Source: CAD feature listing. Evaluate the final solid. Frame: model axes, mm. Coordinates: 2 decimals unless noted, no trailing zeros. Loops run counter-clockwise (first coordinate to the right, second up) from the corner with the lowest first, then second, coordinate; pieces in that order, holes last.
Autodesk Inventor part; units mm, degrees
ref_plane "YZ Plane" through (0, 0, 0) normal (1, 0, 0) x (0, 1, 0)
ref_plane "XZ Plane" through (0, 0, 0) normal (0, 1, 0) x (-1, 0, 0)
ref_plane "XY Plane" through (0, 0, 0) normal (0, 0, 1) x (1, 0, 0)
sketch "Sketch1" plane through (0, 0, 0) normal (0, 0, 1) x (1, 0, 0)
  line L0 (0, 0) -> (10, 0)
  line L1 (10, 0) -> (10, 40)
  line L2 (10, 40) -> (0, 40)
  line L3 (0, 40) -> (0, 0)
  dimension "d0" = 10
  dimension "d1" = 40
extrude "Extrusion1" add sketch "Sketch1" along normal blind 1
sketch "Sketch2" plane through (0, 0, 1) normal (0, 0, 1) x (1, 0, 0)
  line L0 (10, 40) -> (0, 40)
  line L1 (0, 40) -> (5, 40)
  line L2 (5, 40) -> (5, 35)
  circle A0 centre (5, 35) radius 2.5
  line L3 (0, 0) -> (1, 0)
  line L4 (1, 0) -> (5, 0)
  line L5 (0, 0) -> (10, 0)
  line L6 (5, 0) -> (5, 5)
  circle A1 centre (5, 5) radius 2.5
  dimension "d4" = 5
  dimension "d5" = 5
  dimension "d6" = 5
  dimension "d7" = 1
  dimension "d8" = 4
  dimension "d9" = 5
  dimension "d10" = 5
extrude "Extrusion2" cut sketch "Sketch2" against normal blind 1
sketch "Sketch3" plane through (0, 0, 1) normal (0, 0, 1) x (1, 0, 0)
  circle A0 centre (4.7625, 4.7625) radius 4
  point P0 (0, 0)
  dimension "d13" = 8
properties part number "crank"
Q1. Draft query along X for faces 1 (the cylindrical face through (7.385, 35.751, 0.507)), 2 (the flat face through (0, 20.3, 0.5)), 3 (the flat face through (5, 20, 0)). Return one class per face: released by +X, released by -X, zero draft, split by the parting line, or undercut.
Q2. Section query C-C on z = 0.6. Return the cut outline in (x, y), then the cut area to 3 significant figures.
Q3. Section query A-A on x = 5. Return the cut outline in (y, z), then the cut area to 3 significant figures.
Q4. Material intervals for line 1 along Y through (x, z) = (5, 0.6); line 2 along X through (y, z) = (5, 0.55); line 3 along Y through (x, z) = (6, 0.15), sorted ascending.
Q5. First-contact query: pin 1 Ø4 at (x, y) = (5, 5) entering from -Z. Flat tip, straight axial feed; report the tip coordinate or a pass-through.
Q6. Section query B-B on y = 35. Return the cut outline in (x, z), then the cut area to 3 significant figures.
Q7. Section query D-D on y = 6.5. Return the cut outline in (x, z).
Resolved:
1. face 1: undercut
1. face 2: released by -X
1. face 3: zero draft
2. outline: (0, 0) - (10, 0) - (10, 40) - (0, 40) - close; hole circle Ø5 at (5, 5); hole circle Ø5 at (5, 35)
2. area: 361 mm2
3. outline: (0, 0) - (2.5, 0) - (2.5, 1) - (0, 1) - close; (7.5, 0) - (32.5, 0) - (32.5, 1) - (7.5, 1) - close; (37.5, 0) - (40, 0) - (40, 1) - (37.5, 1) - close
3. area: 30.0 mm2
4. line 1: y = 0 to 2.5, 7.5 to 32.5, 37.5 to 40
4. line 2: x = 0 to 2.5, 7.5 to 10
4. line 3: y = 0 to 2.71, 7.29 to 32.71, 37.29 to 40
5. pin 1: passes through
6. outline: (0, 0) - (2.5, 0) - (2.5, 1) - (0, 1) - close; (7.5, 0) - (10, 0) - (10, 1) - (7.5, 1) - close
6. area: 5.00 mm2
7. outline: (0, 0) - (3, 0) - (3, 1) - (0, 1) - close; (7, 0) - (10, 0) - (10, 1) - (7, 1) - close
